from build123d import *

# Parameters (mm, degrees)
BOSS_EXTRUDE1_DEPTH = 3.2
CHAMFER1_SIZE       = 0.5
SKETCH2_R           = 1.625
CUT_EXTRUDE1_DEPTH  = 2


with BuildPart() as part:
    # Sketch1 → Boss-Extrude1 (new body)
    with BuildSketch(Plane(origin=(0, 0, 0), x_dir=(1, 0, 0), z_dir=(0, 1, 0))):
        with BuildLine():
            Line((-17.971705397, 32.627906846), (-13.729256498, 25.279769804))
            ThreePointArc((-13.729256498, 25.279769804), (0, 28.767329478), (13.729256498, 25.279769804))
            Line((13.729256498, 25.279769804), (17.971705397, 32.627906846))
            ThreePointArc((17.971705397, 32.627906846), (0, 37.25), (-17.971705397, 32.627906846))
        make_face()
    extrude(amount=BOSS_EXTRUDE1_DEPTH)

    # Chamfer1
    chamfer1_edges = [part.edges().sort_by_distance(p)[0] for p in [
        (0, 3.2, -28.767329478),
        (15.850480947, 3.2, -28.953838325),
        (0, 3.2, -37.25),
        (15.850480947, 0, -28.953838325),
        (0, 0, -28.767329478),
        (0, 0, -37.25),
        (-15.850480947, 3.2, -28.953838325),
    ]]
    chamfer(chamfer1_edges, length=CHAMFER1_SIZE)

    # Sketch2 → Cut-Extrude1 (cut)
    with BuildSketch(Plane.XZ):
        with Locations(Location((0, -33, 0), (0, 0, 270))):
            Circle(SKETCH2_R)
    extrude(amount=-CUT_EXTRUDE1_DEPTH, mode=Mode.SUBTRACT)


solid = part.part
Check sheet for the modelled part. Datum: model origin and axes. Units: mm. A direction names the side the tool comes from. Round coordinates to 2 decimals unless told otherwise and drop trailing zeros. Loops run counter-clockwise (first coordinate to the right, second up) from the corner with the lowest first, then second, coordinate; pieces in that order, holes last.
1. Sectioned sample at B-B on x = 0. Record the boundary of the cut face in (y, z) (3 decimals), and give its area (3 significant figures).
2. Set-up check for faces 5 (the flat face through (0, 2, -33)), 6 (the flat face through (0, 3.2, -31)): record each of +Z, -Z, +X, -X, +Y, -Y from which the full face is reachable in a straight line by a thin tool's end or side.
3. Mould release check, pull along X, two halves, no side actions. Record for faces 1 (the flat face through (0, 0, -31)), 2 (the flat face through (15.601, 0.247, -29.029)), 3 (the flat face through (-15.661, 2.954, -29.132)), 4 (the conical face through (-0.208, 0.358, -28.909)): released by +X, released by -X, zero draft, split by the parting line, or undercut.
4. Scan lines: probe 1 along X at (y, z) = (1.35, -33) (3 decimals); probe 2 along X at (y, z) = (0.85, -26.25); probe 3 along Y at (x, z) = (0, -32.25). Record each from-to range of solid material in increasing order.
5. Gauge pin test, flat ends, axial feed: pin 1 Ø2.5 at (x, z) = (0, -33) entering from -Y; pin 2 Ø1 at (y, z) = (2, -27.5) entering from +X. Record the tip position at first contact, or that the pin passes through.
6. Sectioned sample at A-A on y = 1.1. Record the boundary of the cut face in (x, z) (3 decimals).
7. Sectioned sample at C-C on z = -30. Record the boundary of the cut face in (x, y).
Recorded:
1. outline: (0, -36.75) - (0.5, -37.25) - (2.7, -37.25) - (3.2, -36.75) - (3.2, -29.267) - (2.7, -28.767) - (0.5, -28.767) - (0, -29.267) - (0, -31.375) - (2, -31.375) - (2, -34.625) - (0, -34.625) - close
1. area: 20.1 mm2
2. face 5: -Y
2. face 6: +Z, -Z, +X, -X, +Y
3. face 1: zero draft
3. face 2: released by +X
3. face 3: released by -X
3. face 4: undercut
4. probe 1: x = -17.279 to -1.625, 1.625 to 17.279
4. probe 2: x = -14.29 to -11.77, 11.77 to 14.29
4. probe 3: y = 2 to 3.2
5. pin 1: stops at y = 2
5. pin 2: stops at x = 15.3
6. outline: (-17.972, -32.628) arc R37.25 ccw to (17.972, -32.628) - (13.729, -25.28) arc R28.767 cw to (-13.729, -25.28) - close; hole circle Ø3.25 at (0, -33)
7. outline: (-16.45, 0) - (15.88, 0) - (16.45, 0.5) - (16.45, 2.7) - (15.88, 3.2) - (-15.88, 3.2) - (-16.45, 2.7) - close
